from build123d import *

# Parameters (mm, degrees)
F0_R     = 1.5
F1_DEPTH = 3
F2_DEPTH = 15
F4_ANGLE = 20


# Not quite as in the source:
# - a feature names something its author has since deleted; it is built from what else it names


with BuildPart() as f1:
    # F0 (on Top) → F1 (new body)
    with BuildSketch(Plane.XY):
        with BuildLine():
            ThreePointArc((4.3e-09, -10), (7.0710678134, -7.0710678103), (10, 0))
            ThreePointArc((10, 0), (7.0710678119, 7.0710678119), (0, 10))
            ThreePointArc((0, 10), (-7.0710678074, 7.0710678163), (-10, 1.26e-08))
            ThreePointArc((-10, 1.26e-08), (-7.0710678148, -7.0710678089), (4.3e-09, -10))
        make_face()
        with BuildLine():
            ThreePointArc((1.5, -8.5), (1.0606601733, -9.5606601703), (4.3e-09, -10))
            ThreePointArc((4.3e-09, -10), (-1.0606601733, -7.4393398297), (1.5, -8.5))
        make_face(mode=Mode.SUBTRACT)
        with BuildLine():
            ThreePointArc((-7, 0), (-8.5000000063, -1.5), (-10, 1.26e-08))
            ThreePointArc((-10, 1.26e-08), (-8.4999999937, 1.5), (-7, 0))
        make_face(mode=Mode.SUBTRACT)
        with BuildLine():
            ThreePointArc((1.4899664426, 1.55), (1.9781213122, 0.842339643), (2.15, 0))
            ThreePointArc((2.15, 0), (-0.842339643, -1.9781213122), (-1.4899664426, 1.55))
            ThreePointArc((-1.4899664426, 1.55), (0, 2.15), (1.4899664426, 1.55))
        make_face(mode=Mode.SUBTRACT)
        with Locations((8.5, 0)):
            Circle(F0_R, mode=Mode.SUBTRACT)
        with BuildLine():
            ThreePointArc((1.5, 8.5), (-1.0606601718, 7.4393398282), (0, 10))
            ThreePointArc((0, 10), (1.0606601718, 9.5606601718), (1.5, 8.5))
        make_face(mode=Mode.SUBTRACT)
        with BuildLine():
            ThreePointArc((-7, 0), (-8.4999999937, 1.5), (-10, 1.26e-08))
            ThreePointArc((-10, 1.26e-08), (-8.5000000063, -1.5), (-7, 0))
        make_face()
        with BuildLine():
            ThreePointArc((1.5, -8.5), (-1.0606601733, -7.4393398297), (4.3e-09, -10))
            ThreePointArc((4.3e-09, -10), (1.0606601733, -9.5606601703), (1.5, -8.5))
        make_face()
        with Locations((8.5, 0)):
            Circle(F0_R)
        with BuildLine():
            ThreePointArc((1.5, 8.5), (1.0606601718, 9.5606601718), (0, 10))
            ThreePointArc((0, 10), (-1.0606601718, 7.4393398282), (1.5, 8.5))
        make_face()
        with BuildLine():
            Line((-1.4899664426, 1.55), (1.4899664426, 1.55))
            ThreePointArc((1.4899664426, 1.55), (0, 2.15), (-1.4899664426, 1.55))
        make_face()
    extrude(amount=F1_DEPTH)

    # F0 (on Top) → F2 (join)
    with BuildSketch(Plane.XY):
        with BuildLine():
            ThreePointArc((1.5, 8.5), (1.0606601718, 9.5606601718), (0, 10))
            ThreePointArc((0, 10), (-1.0606601718, 7.4393398282), (1.5, 8.5))
        make_face()
        with BuildLine():
            ThreePointArc((-7, 0), (-8.4999999937, 1.5), (-10, 1.26e-08))
            ThreePointArc((-10, 1.26e-08), (-8.5000000063, -1.5), (-7, 0))
        make_face()
        with BuildLine():
            ThreePointArc((1.5, -8.5), (-1.0606601733, -7.4393398297), (4.3e-09, -10))
            ThreePointArc((4.3e-09, -10), (1.0606601733, -9.5606601703), (1.5, -8.5))
        make_face()
        with Locations((8.5, 0)):
            Circle(F0_R)
    extrude(amount=F2_DEPTH)


with BuildPart() as f1_1:
    # F4: moved
    add(f1.part.rotate(Axis((0, 0, 24.3583247066), (0, 0, 1)), F4_ANGLE))


solid = f1_1.part
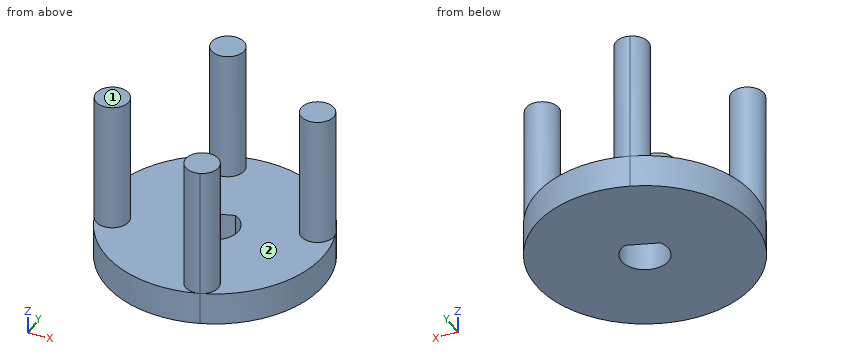
Source: CAD feature listing. Evaluate the final solid. Frame: model axes, mm. Face numbers are marked on the shaded views. A direction names the side the tool comes from. Round coordinates to 2 decimals unless told otherwise and drop trailing zeros. Write each loop counter-clockwise with the first axis right and the second up, starting at its lowest first coordinate (ties: lowest second). Pieces come first, ordered by that corner, then holes. Notation, with made-up numbers: M -27,-28 L -5,-28 A10 ccw -5,-13 Z; hole C 36,30.5 d7. An arc over 180 degrees is marked long. One line per item, written item: value. Start each with the question number.
Item 1: Section query C-C (x = 0). Return the cut outline in (y, z), plus the area to 3 significant figures.
Item 2: Ray query, L1, parallel to X at y = 0, z = 1.65; L2, parallel to Z at x = 1.25, y = 7.5; L3, parallel to X at y = 8, z = 6. Return the intervals inside material, ascending. Write a range as from..to.
Item 3: Section query A-A (z = 10.5). Return the cut outline in (x, y).
Item 4: Set-up query: the marked faces 1 and 2. Return all of +Z, -Z, +X, -X, +Y, -Y with unobstructed straight access to the full face (end or side cutting, diameter ignored); none if empty.
Item 5: Section query B-B (y = 0). Return the cut outline in (x, z).
Item 6: Section query D-D (y = 4). Return the cut outline in (x, z), plus the area to 3 significant figures.
Item 7: Pin query (flat end, axial travel): pin 1 (3 mm diameter, centred on y = -1, z = 9.5, fed in from +X); pin 2 (6 mm diameter, centred on y = 2.5, z = 9.5, fed in from +X); pin 3 (3 mm diameter, centred on x = 5, y = 0, fed in from +Z). Return the tip coordinate at first contact, or that it passes through.
Result set:
1. outline: M -10,0 L -2.15,0 L -2.15,3 L -10,3 Z; M 1.65,0 L 10,0 L 10,3 L 1.65,3 Z
1. area: 48.6 mm²
2. L1: x = -10..-2.15, 2.15..10
2. L2: z = 0..3
2. L3: x = -4.41..-1.41
3. outline: C -7.99,-2.91 d3; C -2.91,7.99 d3; C 2.91,-7.99 d3; C 7.99,2.91 d3
4. face 1: +Z, +X, -X, +Y, -Y
4. face 2: +Z
5. outline: M -10,0 L -2.15,0 L -2.15,3 L -10,3 Z; M 2.15,0 L 10,0 L 10,3 L 2.15,3 Z
6. outline: M -9.17,0 L 9.17,0 L 9.17,3 L 9.01,3 L 9.01,15 L 6.96,15 L 6.96,3 L -9.17,3 Z
6. area: 79.7 mm²
7. pin 1: stops at x = -6.54
7. pin 2: stops at x = 9.49
7. pin 3: stops at z = 3
